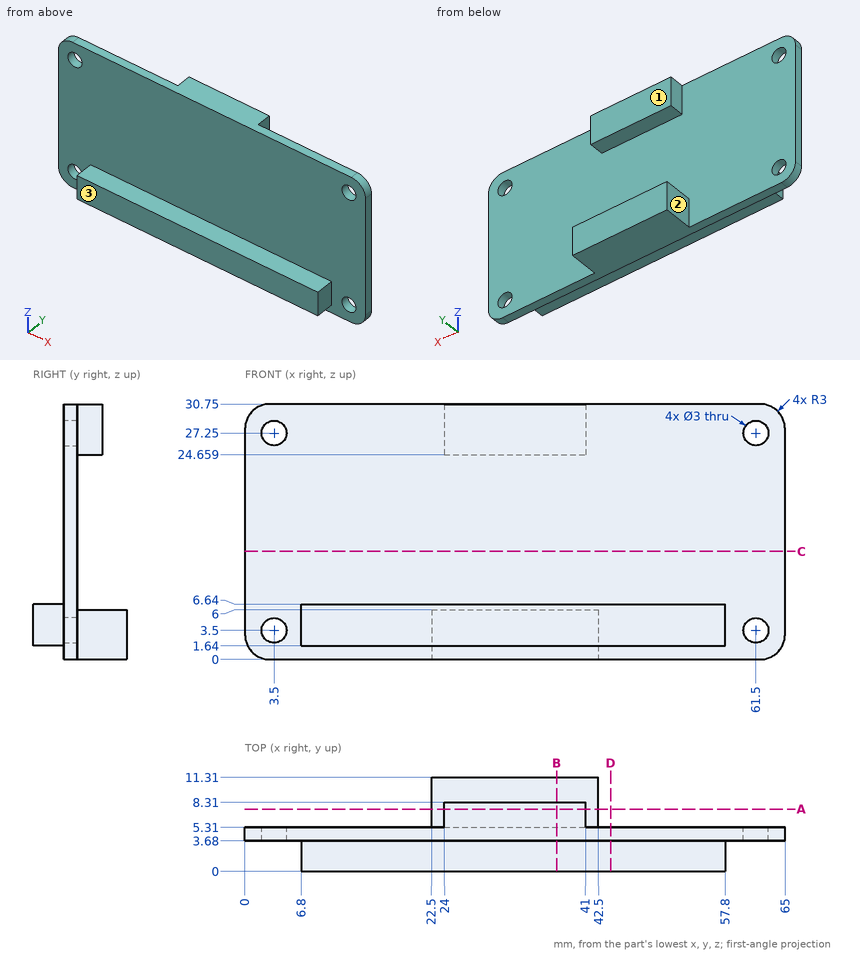
Source: three-view drawing plus pictorial views. Frame: mm from the lowest corner of the part. A direction names the side the tool comes from. Round coordinates to 2 decimals unless told otherwise and drop trailing zeros. Loops run counter-clockwise (first coordinate to the right, second up) from the corner with the lowest first, then second, coordinate; pieces in that order, holes last. Notation, with made-up numbers: (34.5, 7) -> (40.5, 7) arc R16 cw to (40.5, 26) -> close; hole circle Ø8 at (-21.75, 6.25). An arc over 180 degrees is marked (long way). Use one line per item in the form item = value.
Item 1: Cut plane B-B on x = 37.5. Output: boundary loops of the cut face in (y, z).
Evaluation:
outline = (0, 1.64) -> (3.68, 1.64) -> (3.68, 0) -> (11.31, 0) -> (11.31, 6) -> (5.31, 6) -> (5.31, 24.66) -> (8.31, 24.66) -> (8.31, 30.75) -> (3.68, 30.75) -> (3.68, 6.64) -> (0, 6.64) -> close
Item 2: Material intervals for probe 1 along X at (y, z) = (4.6, 3.5); probe 2 along Z at (x, y) = (25, 1.25); probe 3 along Y at (x, z) = (54, 9.5), sorted ascending.
Evaluation:
probe_1 = 0 to 2, 5 to 60, 63 to 65
probe_2 = 1.64 to 6.64
probe_3 = 3.68 to 5.31
Item 3: Cut plane D-D on x = 44. Output: boundary loops of the cut face in (y, z).
Evaluation:
outline = (0, 1.64) -> (3.68, 1.64) -> (3.68, 0) -> (5.31, 0) -> (5.31, 30.75) -> (3.68, 30.75) -> (3.68, 6.64) -> (0, 6.64) -> close
Item 4: Cut plane C-C on z = 13. Output: boundary loops of the cut face in (x, y).
Evaluation:
outline = (0, 3.68) -> (65, 3.68) -> (65, 5.31) -> (0, 5.31) -> close
Item 5: Contact query for flat-ended pins moving along their axis: pin 1 Ø3.5 at (x, z) = (3.5, 3.5) entering from +Y; pin 2 Ø1.8 at (y, z) = (9, 3.5) entering from -X; pin 3 Ø1.8 at (y, z) = (2.5, 3) entering from +X; pin 4 Ø4 at (x, y) = (55.5, 8) entering from +Z. Output: stop coordinate, or through.
Evaluation:
pin_1 = 5.31
pin_2 = 22.5
pin_3 = 57.8
pin_4 = through
Item 6: Cut plane A-A on y = 7.5. Output: boundary loops of the cut face in (x, z).
Evaluation:
outline = (22.5, 0) -> (42.5, 0) -> (42.5, 6) -> (22.5, 6) -> close; (24, 24.66) -> (41, 24.66) -> (41, 30.75) -> (24, 30.75) -> close
Item 7: Access query for the marked faces 1, 2 and 3. Directions: +Z, -Z, +X, -X, +Y, -Y. A direction counts if a zero-diameter tool reaches every point of the face in a straight line with its end or side. Return the directions, or none.
Evaluation:
face_1 = +Z, +X, -X, +Y
face_2 = +Z, -Z, -X, +Y
face_3 = +Z, -Z, +X, -X, -Y
